from build123d import *

# Parameters (mm, degrees)
SKETCH1_W           = 137
SKETCH1_H           = 92
BOSS_EXTRUDE1_DEPTH = 2
SKETCH2_W           = 137
SKETCH2_H           = 92
SKETCH2_W_2         = 133
SKETCH2_H_2         = 88
BOSS_EXTRUDE2_DEPTH = 7
SKETCH3_W           = 137
SKETCH3_H           = 92
SKETCH3_W_2         = 135
SKETCH3_H_2         = 90
BOSS_EXTRUDE3_DEPTH = 2
SKETCH4_R           = 1.35
BOSS_EXTRUDE4_DEPTH = 7
SKETCH8_W           = 108
SKETCH8_H           = 1.9
BOSS_EXTRUDE6_DEPTH = 7
FILLET1_R           = 2
FILLET2_R           = 3
FILLET3_R           = 4
SKETCH11_W          = 108
SKETCH11_H          = 1.9
BOSS_EXTRUDE7_DEPTH = 7
SKETCH12_W          = 97
SKETCH12_H          = 4
CUT_EXTRUDE3_DEPTH  = 2
CUT_EXTRUDE4_START  = -10
SKETCH13_R          = 1.35
CUT_EXTRUDE4_DEPTH  = 10


with BuildPart() as part:
    # Sketch1 → Boss-Extrude1 (new body)
    with BuildSketch(Plane.XY):
        with Locations((68.5, 46)):
            Rectangle(SKETCH1_W, SKETCH1_H)
    extrude(amount=BOSS_EXTRUDE1_DEPTH)

    # Sketch2 → Boss-Extrude2 (add)
    with BuildSketch(Plane.XY.offset(2)):
        with Locations((68.5, 46)):
            Rectangle(SKETCH2_W, SKETCH2_H)
        with Locations((68.5, 46)):
            Rectangle(SKETCH2_W_2, SKETCH2_H_2, mode=Mode.SUBTRACT)
    extrude(amount=BOSS_EXTRUDE2_DEPTH)

    # Sketch3 → Boss-Extrude3 (add)
    with BuildSketch(Plane.XY.offset(9)):
        with Locations((68.5, 46)):
            Rectangle(SKETCH3_W, SKETCH3_H)
        with Locations((68.5, 46)):
            Rectangle(SKETCH3_W_2, SKETCH3_H_2, mode=Mode.SUBTRACT)
    extrude(amount=BOSS_EXTRUDE3_DEPTH)

    # Sketch4 → Boss-Extrude4 (add)
    # profile 1 of 4: a face of its own
    with BuildSketch(Plane.XY.offset(2)):
        with BuildLine():
            Line((7.5, 6), (7.5, 2))
            Line((7.5, 2), (14.5, 2))
            Line((14.5, 2), (14.5, 6))
            ThreePointArc((14.5, 6), (11, 9.5), (7.5, 6))
        make_face()
        with Locations((11, 6)):
            Circle(SKETCH4_R, mode=Mode.SUBTRACT)
    # profile 2 of 4: a face of its own
    with BuildSketch(Plane.XY.offset(2)):
        with BuildLine():
            Line((122.5, 6), (122.5, 2))
            Line((122.5, 2), (129.5, 2))
            Line((129.5, 2), (129.5, 6))
            ThreePointArc((129.5, 6), (126, 9.5), (122.5, 6))
        make_face()
        with Locations((126, 6)):
            Circle(SKETCH4_R, mode=Mode.SUBTRACT)
    # profile 3 of 4: a face of its own
    with BuildSketch(Plane.XY.offset(2)):
        with BuildLine():
            Line((129.5, 86), (129.5, 90))
            Line((129.5, 90), (122.5, 90))
            Line((122.5, 90), (122.5, 86))
            ThreePointArc((122.5, 86), (126, 82.5), (129.5, 86))
        make_face()
        with Locations((126, 86)):
            Circle(SKETCH4_R, mode=Mode.SUBTRACT)
    # profile 4 of 4: a face of its own
    with BuildSketch(Plane.XY.offset(2)):
        with BuildLine():
            Line((14.5, 86), (14.5, 90))
            Line((14.5, 90), (7.5, 90))
            Line((7.5, 90), (7.5, 86))
            ThreePointArc((7.5, 86), (11, 82.5), (14.5, 86))
        make_face()
        with Locations((11, 86)):
            Circle(SKETCH4_R, mode=Mode.SUBTRACT)
    extrude(amount=BOSS_EXTRUDE4_DEPTH)

    # Sketch8 → Boss-Extrude6 (add)
    with BuildSketch(Plane.XY.offset(2)):
        with Locations((68.5, 2.95)):
            Rectangle(SKETCH8_W, SKETCH8_H)
    extrude(amount=BOSS_EXTRUDE6_DEPTH)

    # Fillet1
    fillet1_edges = [part.edges().sort_by_distance(p)[0] for p in [
        (2, 2, 5.5),
        (135, 2, 5.5),
        (135, 90, 5.5),
        (2, 90, 5.5),
    ]]
    fillet(fillet1_edges, radius=FILLET1_R)

    # Fillet2
    fillet2_edges = [part.edges().sort_by_distance(p)[0] for p in [
        (1, 1, 10),
        (136, 1, 10),
        (136, 91, 10),
        (1, 91, 10),
    ]]
    fillet(fillet2_edges, radius=FILLET2_R)

    # Fillet3
    fillet3_edges = [part.edges().sort_by_distance(p)[0] for p in [
        (0, 92, 5.5),
        (137, 92, 5.5),
        (137, 0, 5.5),
        (0, 0, 5.5),
    ]]
    fillet(fillet3_edges, radius=FILLET3_R)

    # Sketch11 → Boss-Extrude7 (add)
    with BuildSketch(Plane.XY.offset(2)):
        with Locations((68.5, 89.05)):
            Rectangle(SKETCH11_W, SKETCH11_H)
    extrude(amount=BOSS_EXTRUDE7_DEPTH)

    # Sketch12 → Cut-Extrude3 (cut)
    with BuildSketch(Plane(origin=(0, 92, 0), x_dir=(1, 0, 0), z_dir=(0, 1, 0))):
        with Locations((73.5, -9)):
            Rectangle(SKETCH12_W, SKETCH12_H)
    extrude(amount=-CUT_EXTRUDE3_DEPTH, mode=Mode.SUBTRACT)

    # Sketch13 → Cut-Extrude4 (cut)
    with BuildSketch(Plane.XY.offset(9).offset(CUT_EXTRUDE4_START)):
        with Locations(Location((11, 86, 0), (0, 0, 180))):
            Circle(SKETCH13_R)
        with Locations(Location((11, 6, 0), (0, 0, 180))):
            Circle(SKETCH13_R)
        with Locations(Location((126, 6, 0), (0, 0, 180))):
            Circle(SKETCH13_R)
        with Locations(Location((126, 86, 0), (0, 0, 180))):
            Circle(SKETCH13_R)
    extrude(amount=CUT_EXTRUDE4_DEPTH, mode=Mode.SUBTRACT)


solid = part.part
Input: part model. Units: mm. Frame: model coordinates. A direction names the side the tool comes from. Coordinates: 2 decimals unless noted, no trailing zeros. Order: outer loops, then holes, each group sorted by start corner. A loop starts at its lowest first (then second) coordinate and runs counter-clockwise, first axis right, second up. Notation, with made-up numbers: M 81,9.5 L 90,9.5 A23 cw 90,35.5 Z; hole C 13.5,73.5 d4. An arc over 180 degrees is marked long. One line per question, with ' | ' between items.
Item 1: Section B-B (y = 22). Output: boundary loops of the cut face in (x, z), then the cut area to 3 significant figures.
Geometry results:
outline: M 0,0 L 137,0 L 137,11 L 136,11 L 136,9 L 135,9 L 135,2 L 2,2 L 2,9 L 1,9 L 1,11 L 0,11 Z | area: 306 mm^2
Item 2: Reachability of faces 1 (the flat face through (131, 90, 5)), 2 (the cylindrical face through (1.141, 90.797, 5.423)) from +Z, -Z, +X, -X, +Y, -Y: full face, straight path, thin tool, end or side. Return the list, or none.
Geometry results:
face 1: +Z | face 2: +Z, -Z, -X, +Y
Item 3: Ray query, line 1 along X through (y, z) = (88, 2.5); line 2 along X through (y, z) = (86, 0.5); line 3 along X through (y, z) = (86, 8.25). Return the intervals inside material, ascending.
Geometry results:
line 1: x = 0 to 2, 7.5 to 14.5, 122.5 to 129.5, 135 to 137 | line 2: x = 0 to 9.65, 12.35 to 124.65, 127.35 to 137 | line 3: x = 0 to 2, 7.5 to 9.65, 12.35 to 14.5, 122.5 to 124.65, 127.35 to 129.5, 135 to 137
Item 4: Section D-D (x = 82). Output: boundary loops of the cut face in (y, z).
Geometry results:
outline: M 0,0 L 92,0 L 92,7 L 90,7 L 90,9 L 88.1,9 L 88.1,2 L 3.9,2 L 3.9,9 L 1,9 L 1,11 L 0,11 Z
Item 5: Section A-A (x = 11). Output: boundary loops of the cut face in (y, z).
Geometry results:
outline: M 0,0 L 4.65,0 L 4.65,9 L 1,9 L 1,11 L 0,11 Z; M 7.35,0 L 84.65,0 L 84.65,9 L 82.5,9 L 82.5,2 L 9.5,2 L 9.5,9 L 7.35,9 Z; M 87.35,0 L 92,0 L 92,11 L 91,11 L 91,9 L 87.35,9 Z
Item 6: Pin query (flat end, axial travel): pin 1 (3.5 mm diameter, centred on x = 11, y = 86, fed in from +Z); pin 2 (8 mm diameter, centred on x = 31, y = 48, fed in from +Z). Return the tip coordinate at first contact, or that it passes through.
Geometry results:
pin 1: stops at z = 9 | pin 2: stops at z = 2
Item 7: Section C-C (z = 4). Give the number of separate pieces and of enclosed holes in the cut face, then the cut area to 3 significant figures.
Geometry results:
separate pieces: 1 | enclosed holes: 5 | area: 1,470 mm^2
Item 8: Draft query along X for faces 3 (the flat face through (68, 88.1, 5)), 4 (the flat face through (137, 45, 5)), 5 (the flat face through (6, 90, 5)), 6 (the cylindrical face through (1.141, 1.203, 5.577)). Return one class per face: released by +X, released by -X, zero draft, split by the parting line, or undercut.
Geometry results:
face 3: undercut | face 4: released by +X | face 5: undercut | face 6: released by -X
